Autodesk Inventor part; units mm, degrees
ref_plane "YZ Plane" through (0, 0, 0) normal (1, 0, 0) x (0, 1, 0)
ref_plane "XZ Plane" through (0, 0, 0) normal (0, 1, 0) x (-1, 0, 0)
ref_plane "XY Plane" through (0, 0, 0) normal (0, 0, 1) x (1, 0, 0)
sketch "Эскиз1" plane through (0, 0, 0) normal (0, 0, 1) x (1, 0, 0)
  line L0 (18, -18) -> (-12, -18)
  line L1 (-12, -18) -> (-12, 18)
  line L2 (-12, 18) -> (18, 18)
  line L3 (18, 18) -> (18, -18)
  circle A0 centre (0, 0) radius 6.25
  dimension "d0" = 36
  dimension "d1" = 12.5
  dimension "d5" = 18
  dimension "d6" = 12
  dimension "d8" = 30
extrude "Выдавливание1" add sketch "Эскиз1" along normal blind 5
fillet "Сопряжение1" radius 2 4 edges at (-12, -18, 2.5) (-12, 18, 2.5) (18, 18, 2.5) (18, -18, 2.5)
properties part number "платик под редуктор"
Can you work these out from the model? Positions are in its coordinate system, mm. Round coordinates to 2 decimals unless told otherwise and drop trailing zeros. Loops run counter-clockwise (first coordinate to the right, second up) from the corner with the lowest first, then second, coordinate; pieces in that order, holes last. Notation, with made-up numbers: (-28.5, 42.5) -> (-8.5, 42.5) arc R13 cw to (-8.5, 67.5) -> close; hole circle Ø4 at (82, 37.5). An arc over 180 degrees is marked (long way). One line per item, written item: value. Start each with the question number.
1. If we section it at C-C, the plane y = 0: Write out the boundary of the cut face in (x, z), then the cut area to 3 significant figures.
2. If we section it at A-A, the plane x = 0: Write out the boundary of the cut face in (y, z).
3. If I drill on probe 1 along Y at (x, z) = (0, 1.9); probe 2 along X at (y, z) = (-4, 4.55); probe 3 along X at (y, z) = (-1, 3.9), over which ranges is the centre line in solid material (lowest first)?
4. If we mould it in two halves opening along Y, with no side actions, what happens to faces 1 (the flat face through (3, 18, 2)), 2 (the flat face through (3, -18, 2)), 3 (the cylindrical face through (5.96, -1.88, 2.46))? For each: pulls with the +Y half, pulls with the -Y half, needs draft (parallel to the pull), parting line crosses it, or undercut.
5. If we section it at B-B, the plane z = 1.9: Write out the boundary of the cut face in (x, y).
Calculated:
1. outline: (-12, 0) -> (-6.25, 0) -> (-6.25, 5) -> (-12, 5) -> close; (6.25, 0) -> (18, 0) -> (18, 5) -> (6.25, 5) -> close
1. area: 87.5 mm²
2. outline: (-18, 0) -> (-6.25, 0) -> (-6.25, 5) -> (-18, 5) -> close; (6.25, 0) -> (18, 0) -> (18, 5) -> (6.25, 5) -> close
3. probe 1: y = -18 to -6.25, 6.25 to 18
3. probe 2: x = -12 to -4.8, 4.8 to 18
3. probe 3: x = -12 to -6.17, 6.17 to 18
4. face 1: pulls with the +Y half
4. face 2: pulls with the -Y half
4. face 3: undercut
5. outline: (-12, -16) arc R2 ccw to (-10, -18) -> (16, -18) arc R2 ccw to (18, -16) -> (18, 16) arc R2 ccw to (16, 18) -> (-10, 18) arc R2 ccw to (-12, 16) -> close; hole circle Ø12.5 at (0, 0)
